Input: part model. Units: mm. Frame: model coordinates. Give positions to 0.01 mm unless a question says otherwise; leave off trailing zeros. Loops run counter-clockwise (first coordinate to the right, second up) from the corner with the lowest first, then second, coordinate; pieces in that order, holes last. Notation, with made-up numbers: M 19.25,42 L 78.25,42 A28 cw 78.25,67 Z; hole C -1,50.25 d1. An arc over 180 degrees is marked long. One line per item, written item: value. Start each with the question number.
(1) Section C-C on z = 0.9. Output: boundary loops of the cut face in (x, y), plus the area to 3 significant figures.
(2) Section A-A on y = -4.5. Output: boundary loops of the cut face in (x, z).
(3) Section B-B on x = 0. Output: boundary loops of the cut face in (y, z), plus the area to 3 significant figures.
(4) Ray query, line 1 along Y through (x, z) = (-18, 0.7); line 2 along Y through (x, z) = (1.5, 1.9); line 3 along X through (y, z) = (0.5, 1.45). Return the intervals inside material, ascending. Write a range as from..to.
Autodesk Inventor part; units mm, degrees
ref_plane "YZ Plane" through (0, 0, 0) normal (1, 0, 0) x (0, 1, 0)
ref_plane "XZ Plane" through (0, 0, 0) normal (0, 1, 0) x (-1, 0, 0)
ref_plane "XY Plane" through (0, 0, 0) normal (0, 0, 1) x (1, 0, 0)
sketch "Boceto1" plane through (0, 0, 0) normal (0, 0, 1) x (1, 0, 0)
  line L0 (-27.5, -12.5) -> (27.5, -12.5)
  line L1 (27.5, -12.5) -> (27.5, 12.5)
  line L2 (27.5, 12.5) -> (-27.5, 12.5)
  line L3 (-27.5, 12.5) -> (-27.5, -12.5)
  line L4 (-27.5, -12.5) -> (27.5, 12.5) construction
  line L5 (27.5, -12.5) -> (-27.5, 12.5) construction
  circle A0 centre (0, 0) radius 2
  circle A1 centre (0, -4.5) radius 0.75
  circle A2 centre (0, 4.5) radius 0.75
  circle A3 centre (4.5, 0) radius 0.75
  circle A4 centre (-4.5, 0) radius 0.75
  line L6 (0, 0) -> (18, 0) construction
  line L7 (0, 0) -> (18, 0) construction
  circle A5 centre (-18, 0) radius 0.75
  circle A6 centre (18, 0) radius 0.75
  dimension "d0" = 55
  dimension "d1" = 25
  dimension "d2" = 4
  dimension "d4" = 1.5
  dimension "d8" = 1.5
  dimension "d9" = 1.5
  dimension "d10" = 1.5
  dimension "d15" = 1.5
  dimension "d16" = 1.5
extrude "Extrusión1" add sketch "Boceto1" along normal blind 2
sketch "Boceto2" plane through (0, 0, 0) normal (1, 0, 0) x (0, 1, 0)
  point P0 (-12.5, 0)
sketch "Boceto3" plane through (0, 0, 2) normal (0, 0, 1) x (1, 0, 0)
  point P0 (0, 0)
properties part number "frontal" material "Acero, galvanizado"
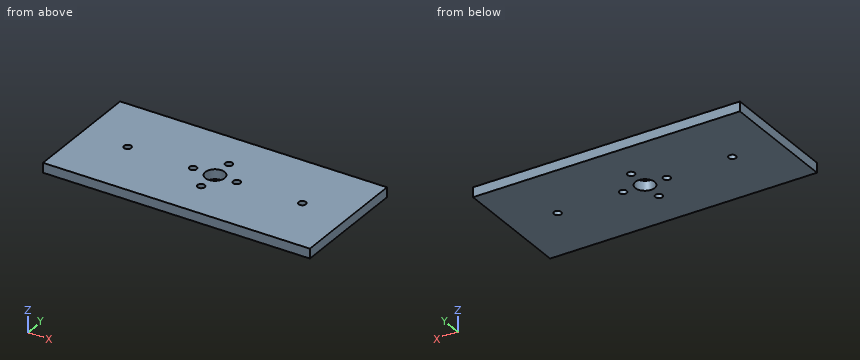
Output values:
1. outline: M -27.5,-12.5 L 27.5,-12.5 L 27.5,12.5 L -27.5,12.5 Z; hole C -18,0 d1.5; hole C -4.5,0 d1.5; hole C 0,0 d4; hole C 0,-4.5 d1.5; hole C 0,4.5 d1.5; hole C 4.5,0 d1.5; hole C 18,0 d1.5
1. area: 1,350 mm²
2. outline: M -27.5,0 L -0.75,0 L -0.75,2 L -27.5,2 Z; M 0.75,0 L 27.5,0 L 27.5,2 L 0.75,2 Z
3. outline: M -12.5,0 L -5.25,0 L -5.25,2 L -12.5,2 Z; M -3.75,0 L -2,0 L -2,2 L -3.75,2 Z; M 2,0 L 3.75,0 L 3.75,2 L 2,2 Z; M 5.25,0 L 12.5,0 L 12.5,2 L 5.25,2 Z
3. area: 36.0 mm²
4. line 1: y = -12.5..-0.75, 0.75..12.5
4. line 2: y = -12.5..-1.32, 1.32..12.5
4. line 3: x = -27.5..-18.56, -17.44..-5.06, -3.94..-1.94, 1.94..3.94, 5.06..17.44, 18.56..27.5
